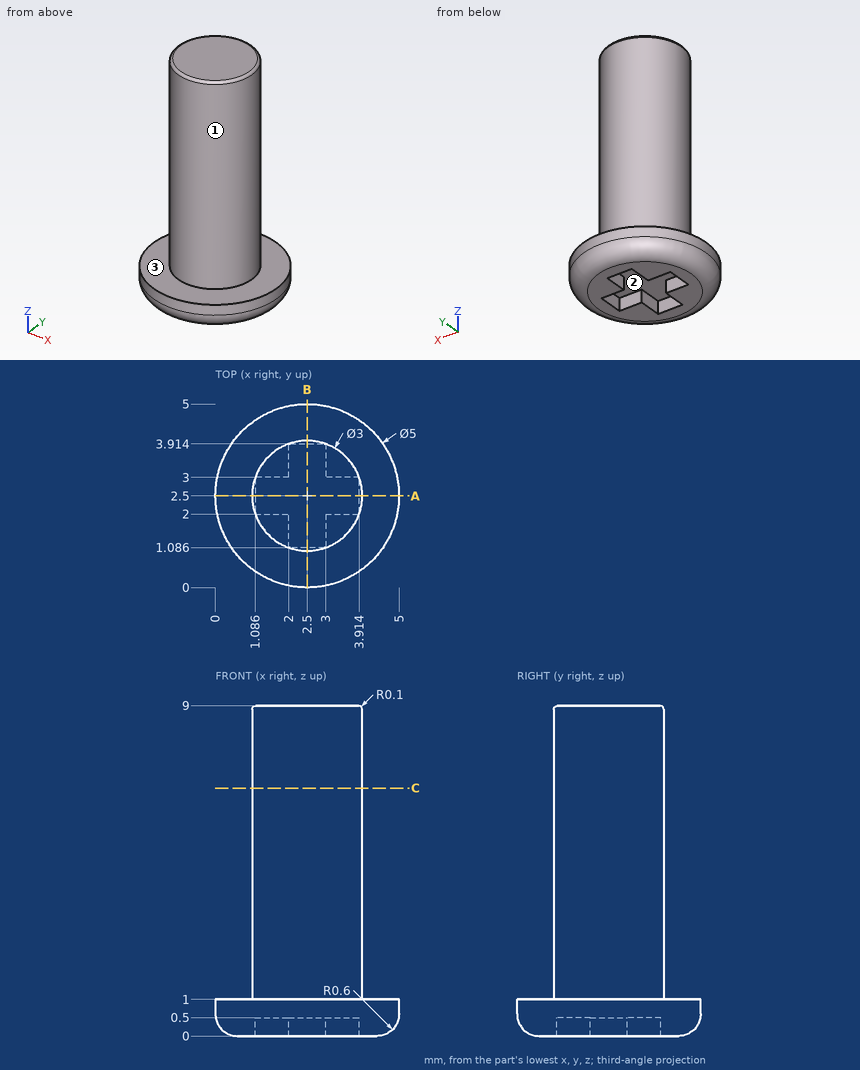
Check sheet for the drawn part. Datum: minimum x, y, z corner. Units: mm. Round coordinates to 2 decimals unless told otherwise and drop trailing zeros. Order: outer loops, then holes, each group sorted by start corner. A loop starts at its lowest first (then second) coordinate and runs counter-clockwise, first axis right, second up. Notation, with made-up numbers: (-38, 70) - (15, 70) arc R30 cw to (15, 107) - close; hole circle Ø9 at (20.5, -14). An arc over 180 degrees is marked (long way). Use a Markdown table: item, result. Add a question column.
(1) Sectioned sample at C-C, the plane z = 6.75. Enter the section's corners in (x, y).
(2) Sectioned sample at A-A, the plane y = 2.5. Enter the section's corners in (x, z).
(3) Material ranges on line 1 along Z through (x, y) = (2.75, 3.1); line 2 along X through (y, z) = (0.45, 0.5) (1 decimal); line 3 along Z through (x, y) = (0.3, 3.1) (1 decimal), recorded low to high. Write a range as [from, to].
(4) Release check for a two-part mould opening along Y. For the marked faces 1, 2 and 3 record: pulls with the +Y half, pulls with the -Y half, needs draft (parallel to the pull), parting line crosses it, or undercut.
(5) Depth check by flat-ended pin: pin 1 (2 mm diameter, centred on y = 0.5, z = 3, fed in from +X); pin 2 (0.8 mm diameter, centred on x = 2, y = 2, fed in from -Z); pin 3 (3 mm diameter, centred on y = 4, z = 6.5, fed in from +X); pin 4 (1 mm diameter, centred on x = 4, z = 7.5, fed in from -Y). Enter the tip coordinate at first touch or a pass-through.
Answers below:
| question | item | result |
|---|---|---|
| 1 | outline | circle Ø3 at (2.5, 2.5) |
| 2 | outline | (0, 0.6) arc R0.6 ccw to (0.6, 0) - (1.09, 0) - (1.09, 0.5) - (3.91, 0.5) - (3.91, 0) - (4.4, 0) arc R0.6 ccw to (5, 0.6) - (5, 1) - (4, 1) - (4, 8.9) arc R0.1 ccw to (3.9, 9) - (1.1, 9) arc R0.1 ccw to (1, 8.9) - (1, 1) - (0, 1) - close |
| 3 | line 1 | [0.5, 9] |
| 3 | line 2 | [1.1, 3.9] |
| 3 | line 3 | [0.1, 1] |
| 4 | face 1 | parting line crosses it |
| 4 | face 2 | undercut |
| 4 | face 3 | needs draft |
| 5 | pin 1 | x = 3.62 |
| 5 | pin 2 | z = 0 |
| 5 | pin 3 | x = 4 |
| 5 | pin 4 | y = 1.38 |
